The model under review builds one solid part; all positions refer to its coordinate system, in mm. Face numbers are marked on the shaded views. A direction names the side the tool comes from. Round coordinates to 2 decimals unless told otherwise and drop trailing zeros. Write each loop counter-clockwise with the first axis right and the second up, starting at its lowest first coordinate (ties: lowest second). Pieces come first, ordered by that corner, then holes. Notation, with made-up numbers: (-34, 88.5) - (-2, 88.5) arc R23 ccw to (-2, 99.5) - close; hole circle Ø10 at (31, 67.5). An arc over 180 degrees is marked (long way). Return JSON: item names as keys, results as strings.
from build123d import *

# Parameters (mm, degrees)
F0_R     = 6.35
F1_DEPTH = 25.4
F2_W     = 61.6878718138
F2_H     = 34.2521034181
F3_DEPTH = 25.4
F5_DEPTH = 36.322
F6_R     = 3.81
F7_DEPTH = 12.7
F8_R     = 3.81
F9_DEPTH = 12.7


with BuildPart() as f1:
    # F0 (on Top) → F1 (new body)
    with BuildSketch(Plane.XY):
        with BuildLine():
            Line((48.9668589424, 24.4255484226), (-48.9668589424, 24.4255484226))
            ThreePointArc((-48.9668589424, 24.4255484226), (-73.5081685676, -0.1157612025), (-48.9668589424, -24.6570708277))
            Line((-48.9668589424, -24.6570708277), (48.9668589424, -24.6570708277))
            ThreePointArc((48.9668589424, -24.6570708277), (73.5081685676, -0.1157612025), (48.9668589424, 24.4255484226))
        make_face()
        with Locations((-48.9668589424, 0)):
            Circle(F0_R, mode=Mode.SUBTRACT)
        with Locations((48.9668589424, 0)):
            Circle(F0_R, mode=Mode.SUBTRACT)
    extrude(amount=F1_DEPTH)

    # F2 (on face) → F3 (join)
    with BuildSketch(Plane.XY.offset(25.4)):
        with Locations((-1.2954026461, -0.45302324)):
            Rectangle(F2_W, F2_H)
    extrude(amount=F3_DEPTH)

    # F4 (on face) → F5 (cut)
    with BuildSketch(Plane.XZ.offset(17.579074949)):
        with BuildLine():
            Line((16.8485332608, 50.8), (-19.439338553, 50.8))
            Line((-19.439338553, 50.8), (-19.439338553, 37.702742964))
            ThreePointArc((-19.439338553, 37.702742964), (-1.2954026461, 27.2985841975), (16.8485332608, 37.702742964))
            Line((16.8485332608, 37.702742964), (16.8485332608, 50.8))
        make_face()
    extrude(amount=-F5_DEPTH, mode=Mode.SUBTRACT)

    # F6 (on face) → F7 (join)
    with BuildSketch(Plane(origin=(-32.139338553, 0, 0), x_dir=(0, -1, 0), z_dir=(-1, 0, 0))):
        with BuildLine():
            Line((-16.6730284691, 50.8), (17.579074949, 50.8))
            ThreePointArc((17.579074949, 50.8), (0.45302324, 63.5928311153), (-16.6730284691, 50.8))
        make_face()
        with Locations((0, 56.2153086066)):
            Circle(F6_R, mode=Mode.SUBTRACT)
    extrude(amount=-F7_DEPTH)

    # F8 (on face) → F9 (join)
    with BuildSketch(Plane.YZ.offset(29.5485332608)):
        with BuildLine():
            ThreePointArc((16.6730284691, 50.8), (-0.45302324, 63.5665881357), (-17.579074949, 50.8))
            Line((-17.579074949, 50.8), (16.6730284691, 50.8))
        make_face()
        with Locations((-0.45302324, 56.8834878504)):
            Circle(F8_R, mode=Mode.SUBTRACT)
    extrude(amount=-F9_DEPTH)


solid = f1.part
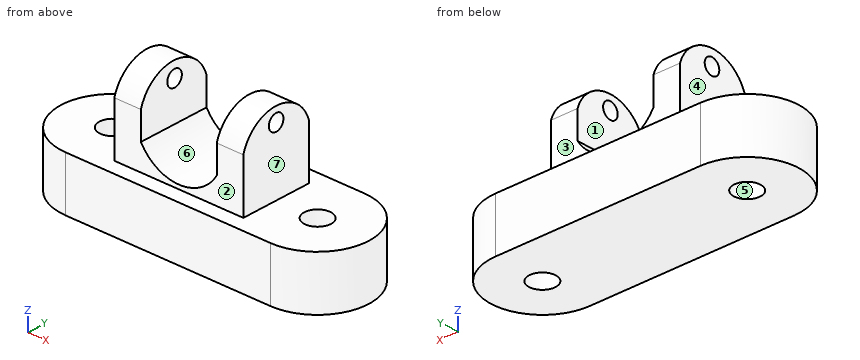
(1) Add section D-D (y = 8.5). Write out the cut boundary in (x, z).
Filled in:
{"outline": "(-71.95, 0) - (71.95, 0) - (71.95, 25.4) - (29.55, 25.4) - (29.55, 61.16) - (16.85, 61.16) - (16.85, 37.7) arc R21.02 cw to (-19.44, 37.7) - (-19.44, 61.19) - (-32.14, 61.19) - (-32.14, 25.4) - (-71.95, 25.4) - close"}
(2) For the marked faces 1, 2 and 3, list the 3-axis set-ups (+Z, -Z, +X, -X, +Y, -Y) from which the entire face can be reached by the end or side of a thin tool; tool diameter is ignored.
Filled in:
{"face 1": "+Z, +Y, -Y", "face 2": "+Z, +X, -X, -Y", "face 3": "+Z, +X, -X, +Y"}
(3) Wall thickness on line 1 (X direction, y = 8.5, z = 38); line 2 (Z direction, x = 47, y = 10.5); line 3 (X direction, y = 7.5, z = 37.5): over which ranges is each line inside the solid? List them lowest first.
Filled in:
{"line 1": "x = -32.14 to -19.44, 16.85 to 29.55", "line 2": "z = 0 to 25.4", "line 3": "x = -32.14 to -19.32, 16.73 to 29.55"}
(4) Mouldability with a two-part tool opening along X and no side actions: class the marked faces 4, 5, 6 and 7 as released by +X, released by -X, zero draft, split by the parting line, or undercut.
Filled in:
{"face 4": "released by -X", "face 5": "undercut", "face 6": "undercut", "face 7": "released by +X"}
(5) Add section A-A (z = 45). Write out the cut boundary in (x, y).
Filled in:
{"outline": "(-32.14, -17.58) - (-19.44, -17.58) - (-19.44, 16.67) - (-32.14, 16.67) - close; (16.85, -17.58) - (29.55, -17.58) - (29.55, 16.67) - (16.85, 16.67) - close"}
(6) Clearance check with flat-ended pins moving along their axes: pin 1 Ø12 at (x, y) = (16.5, -10) entering from +Z; pin 2 Ø12.5 at (x, z) = (0.5, 35.5) entering from -Y; pin 3 Ø10 at (y, z) = (-7, 47) entering from +X; pin 4 Ø12 at (x, y) = (-29.5, 3.5) entering from -Z. State where each tip first meets the part, or that it passes through.
Filled in:
{"pin 1": "stops at z = 63.21", "pin 2": "passes through", "pin 3": "stops at x = 29.55", "pin 4": "stops at z = 0"}
(7) Add section C-C (x = -30). Write out the cut boundary in (y, z), plus the area to 3 significant figures.
Filled in:
{"outline": "(-24.66, 0) - (24.43, 0) - (24.43, 25.4) - (16.67, 25.4) - (16.67, 50.8) arc R17.86 ccw to (-17.58, 50.8) - (-17.58, 25.4) - (-24.66, 25.4) - close; hole circle Ø7.62 at (0, 56.22)", "area": "2,390 mm2"}
(8) Add section B-B (y = 0). Write out the cut boundary in (x, z).
Filled in:
{"outline": "(-73.51, 0) - (-55.32, 0) - (-55.32, 25.4) - (-73.51, 25.4) - close; (-42.62, 0) - (42.62, 0) - (42.62, 25.4) - (29.55, 25.4) - (29.55, 53.1) - (16.85, 53.1) - (16.85, 37.7) arc R21.02 cw to (-19.44, 37.7) - (-19.44, 52.41) - (-32.14, 52.41) - (-32.14, 25.4) - (-42.62, 25.4) - close; (-32.14, 60.03) - (-19.44, 60.03) - (-19.44, 63.59) - (-32.14, 63.59) - close; (16.85, 60.67) - (29.55, 60.67) - (29.55, 63.56) - (16.85, 63.56) - close; (55.32, 0) - (73.51, 0) - (73.51, 25.4) - (55.32, 25.4) - close"}
